Input: part model. Units: mm. Frame: model coordinates. A direction names the side the tool comes from. Coordinates: 2 decimals unless noted, no trailing zeros. Loops run counter-clockwise (first coordinate to the right, second up) from the corner with the lowest first, then second, coordinate; pieces in that order, holes last.
(1) Section D-D, the plane x = 79. Return loops of the section in (y, z), then the cut area to 3 significant figures.
(2) Set-up query: faces 1 (the face through (94.808, -5.535, -0.189)), 2 (the face through (23, -2, 5)), 3 (the face through (33.98, -2.465, -20.944)). Return all of +Z, -Z, +X, -X, +Y, -Y with unobstructed straight access to the full face (end or side cutting, diameter ignored); none if empty.
(3) Section C-C, the plane z = -21.5. Return loops of the section in (x, y), then the cut area to 3 significant figures.
(4) Contact query for flat-ended pins moving along their axis: P1, Ø4, axis at x = -43.5, z = -16, coming from the -Y side; P2, Ø9, axis at x = 43, z = 0, coming from the -Y side; P3, Ø3, axis at y = -5.5, z = -5.5, coming from the +X side. Output: stop coordinate, or through.
(5) Line query: L1, parallel to X at y = -1.75, z = 0; L2, parallel to Z at x = -39.5, y = -2.25; L3, parallel to X at y = -3.5, z = 4. Output: solid intervals per line, ascending.
(6) Section A-A, the plane x = -43.5. Return loops of the section in (y, z).
(7) Section B-B, the plane x = 43. Return loops of the section in (y, z).
(8) Mould query, pull axis Z, two halves, no side actions, for faces 4 (the face through (107, -8, 7)), 5 (the face through (46.966, -1.479, 0.521)), 6 (the face through (53.344, -6.972, -13.491)). Classes: released by +Z, released by -Z, zero draft, split by the parting line, or undercut.
```python
from build123d import *

# Parameters (mm, degrees)
SKETCH28_R           = 5
SKETCH28_R_2         = 4
SKETCH28_R_3         = 1.55
SKETCH28_W           = 10
SKETCH28_H           = 3
BOSS_EXTRUDE10_DEPTH = 5
SKETCH25_R           = 17
BOSS_EXTRUDE8_DEPTH  = 3
SKETCH30_R           = 17
BOSS_EXTRUDE11_DEPTH = 4
SKETCH32_R           = 9.7
CUT_EXTRUDE3_DEPTH   = 6
SKETCH33_R           = 8.2
CUT_EXTRUDE4_DEPTH   = 5


with BuildPart() as part:
    # Sketch28 → Boss-Extrude10 (new body)
    with BuildSketch(Plane(origin=(-32, 0, 0), x_dir=(0, 0, 1), z_dir=(0, -1, 0))):
        with BuildLine():
            Line((-25, 15), (25, 15))
            Line((25, 15), (25, 5))
            Line((25, 5), (17, -135))
            ThreePointArc((17, -135), (0, -152), (-17, -135))
            Line((-17, -135), (-25, 5))
            Line((-25, 5), (-25, 15))
        make_face()
        with Locations(Location((0, -135, 0), (0, 0, 180))):
            Circle(SKETCH28_R, mode=Mode.SUBTRACT)
        with Locations(Location((0, -75, 0), (0, 0, 180))):
            Circle(SKETCH28_R_2, mode=Mode.SUBTRACT)
        with Locations(Location((8, 8.5, 0), (0, 0, 180))):
            Circle(SKETCH28_R_3, mode=Mode.SUBTRACT)
        with Locations(Location((-8, 8.5, 0), (0, 0, 180))):
            Circle(SKETCH28_R_3, mode=Mode.SUBTRACT)
        with Locations(Location((16, 11.5, 0), (0, 0, 180))):
            Circle(SKETCH28_R_3, mode=Mode.SUBTRACT)
        with Locations(Location((-16, 11.5, 0), (0, 0, 180))):
            Circle(SKETCH28_R_3, mode=Mode.SUBTRACT)
        with Locations(Location((-15.5, -56.5, 0), (0, 0, 180))):
            Circle(SKETCH28_R_3, mode=Mode.SUBTRACT)
        with Locations(Location((15.5, -56.5, 0), (0, 0, 180))):
            Circle(SKETCH28_R_3, mode=Mode.SUBTRACT)
        with Locations((0, -55)):
            Rectangle(SKETCH28_W, SKETCH28_H, mode=Mode.SUBTRACT)
    extrude(amount=BOSS_EXTRUDE10_DEPTH)

    # Sketch25 → Boss-Extrude8 (add)
    with BuildSketch(Plane(origin=(0, -5, 0), x_dir=(0, 0, 1), z_dir=(0, -1, 0))):
        with Locations((0, -103)):
            Circle(SKETCH25_R)
    extrude(amount=BOSS_EXTRUDE8_DEPTH)

    # Sketch30 → Boss-Extrude11 (add)
    with BuildSketch(Plane(origin=(0, -5, 0), x_dir=(0, 0, 1), z_dir=(0, -1, 0))):
        with Locations((0, -43)):
            Circle(SKETCH30_R)
    extrude(amount=BOSS_EXTRUDE11_DEPTH)

    # Sketch32 → Cut-Extrude3 (cut)
    with BuildSketch(Plane.XZ.offset(9)):
        with Locations((43, 0)):
            Circle(SKETCH32_R)
    extrude(amount=-CUT_EXTRUDE3_DEPTH, mode=Mode.SUBTRACT)

    # Sketch33 → Cut-Extrude4 (cut)
    with BuildSketch(Plane.XZ.offset(8)):
        with Locations((103, -0.549344368)):
            Circle(SKETCH33_R)
    extrude(amount=-CUT_EXTRUDE4_DEPTH, mode=Mode.SUBTRACT)


solid = part.part
```
Report:
1. outline: (-5, -18.37) - (0, -18.37) - (0, 18.37) - (-5, 18.37) - close
1. area: 184 mm2
2. face 1: -Y
2. face 2: +Y, -Y
2. face 3: -Z, +X, +Y, -Y
3. outline: (-47, -5) - (24.25, -5) - (24.25, 0) - (-47, 0) - close
3. area: 356 mm2
4. P1: stops at y = -5
4. P2: stops at y = -3
4. P3: stops at x = 119.52
5. L1: x = -47 to 21.5, 24.5 to 39, 47 to 98, 108 to 120
5. L2: z = -25 to -9.18, -6.82 to 6.82, 9.18 to 25
5. L3: x = -47 to 21.5, 24.5 to 34.16, 51.84 to 96.18, 109.82 to 119.52
6. outline: (-5, -25) - (0, -25) - (0, -17.55) - (-5, -17.55) - close; (-5, -14.45) - (0, -14.45) - (0, 14.45) - (-5, 14.45) - close; (-5, 17.55) - (0, 17.55) - (0, 25) - (-5, 25) - close
7. outline: (-9, -17) - (-5, -17) - (-5, -20.43) - (0, -20.43) - (0, -4) - (-3, -4) - (-3, -9.7) - (-9, -9.7) - close; (-9, 9.7) - (-3, 9.7) - (-3, 4) - (0, 4) - (0, 20.43) - (-5, 20.43) - (-5, 17) - (-9, 17) - close
8. face 4: zero draft
8. face 5: undercut
8. face 6: split by the parting line
